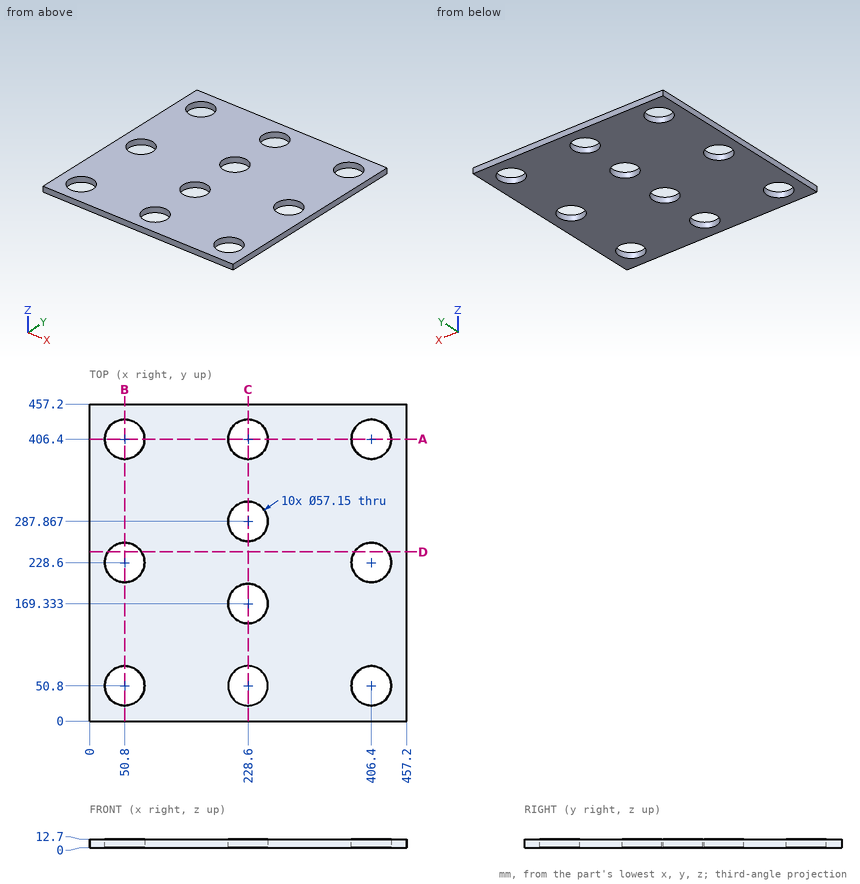
The drawing under review shows one solid part. Ordinate dimensions are in mm from its lowest x, y, z. Coordinates: 2 decimals unless noted, no trailing zeros. Loops run counter-clockwise (first coordinate to the right, second up) from the corner with the lowest first, then second, coordinate; pieces in that order, holes last. Notation, with made-up numbers: (40.5, -15.5) - (92.5, -15.5) arc R16 ccw to (92.5, 11.5) - close; hole circle Ø3 at (71, 82). An arc over 180 degrees is marked (long way). Return JSON: item names as keys, results as strings.
Item 1: Take a section at A-A (y = 406.4). Give the boundary of the cut face in (x, z) (1 decimal).
Determined:
{"outline": "(0, 0) - (22.2, 0) - (22.2, 12.7) - (0, 12.7) - close; (79.4, 0) - (200, 0) - (200, 12.7) - (79.4, 12.7) - close; (257.2, 0) - (377.8, 0) - (377.8, 12.7) - (257.2, 12.7) - close; (435, 0) - (457.2, 0) - (457.2, 12.7) - (435, 12.7) - close"}
Item 2: Take a section at D-D (y = 244). Give the boundary of the cut face in (x, z).
Determined:
{"outline": "(0, 0) - (26.73, 0) - (26.73, 12.7) - (0, 12.7) - close; (74.87, 0) - (382.33, 0) - (382.33, 12.7) - (74.87, 12.7) - close; (430.47, 0) - (457.2, 0) - (457.2, 12.7) - (430.47, 12.7) - close"}
Item 3: For line 1 (X direction, y = 228.6, z = 7.25) (1 decimal); line 2 (Y direction, x = 228.6, z = 3.25) (1 decimal); line 3 (X direction, y = 406.4, z = 3.75) (1 decimal), list the stretches that pass through material, from the lowest coordinate up.
Determined:
{"line 1": "x = 0 to 22.2, 79.4 to 377.8, 435 to 457.2", "line 2": "y = 0 to 22.2, 79.4 to 140.8, 197.9 to 259.3, 316.4 to 377.8, 435 to 457.2", "line 3": "x = 0 to 22.2, 79.4 to 200, 257.2 to 377.8, 435 to 457.2"}
Item 4: Insertion check: pin 1 (3 mm diameter, centred on x = 74, y = 111, fed in from -Z). The pin has a flat end and moves straight along its axis. Give the tip position at first contact, or say it passes through.
Determined:
{"pin 1": "stops at z = 0"}
Item 5: Take a section at C-C (x = 228.6). Give the boundary of the cut face in (y, z) (1 decimal), then the cut area to 3 significant figures.
Determined:
{"outline": "(0, 0) - (22.2, 0) - (22.2, 12.7) - (0, 12.7) - close; (79.4, 0) - (140.8, 0) - (140.8, 12.7) - (79.4, 12.7) - close; (197.9, 0) - (259.3, 0) - (259.3, 12.7) - (197.9, 12.7) - close; (316.4, 0) - (377.8, 0) - (377.8, 12.7) - (316.4, 12.7) - close; (435, 0) - (457.2, 0) - (457.2, 12.7) - (435, 12.7) - close", "area": "2,900 mm2"}
